Geometry check sheet. Reference: the model listing, model coordinates, mm. Face numbers are marked on the shaded views. A direction names the side the tool comes from. Coordinates: 2 decimals unless noted, no trailing zeros. Write each loop counter-clockwise with the first axis right and the second up, starting at its lowest first coordinate (ties: lowest second). Pieces come first, ordered by that corner, then holes. Notation, with made-up numbers: (33, 33) -> (57, 33) arc R22 ccw to (57, 51) -> close; hole circle Ø3 at (-23.75, 21.5). An arc over 180 degrees is marked (long way). Answer in a Markdown table with one row per item. Add a question column.
Q1. Thickness scan on line 1 (X direction, y = 8.25, z = 4.5); line 2 (Y direction, x = -15.5, z = 5.25); line 3 (Y direction, x = -9.75, z = 5.75). Record the ranges inside material, lowest first.
Q2. Section check D-D, the plane x = -22.75. Record the boundary of the cut face in (y, z).
Q3. Section check A-A, the plane y = 8. Record the boundary of the cut face in (x, z), and give its area (3 significant figures).
Q4. Section check B-B, the plane x = -6. Record the boundary of the cut face in (y, z), and give its area (3 significant figures).
Q5. Tool access check on the marked faces 1, 2 and 3. Record the directions out of +Z, -Z, +X, -X, +Y, -Y that give a thin tool (end or side, any length) a straight path to the whole face; none if there is none.
Q6. Section check C-C, the plane z = 2. Record the boundary of the cut face in (x, y).
Q7. Release check for a two-part mould opening along Z. For the marked faces 4, 5 and 6 record: pulls with the +Z half, pulls with the -Z half, needs draft (parallel to the pull), parting line crosses it, or undercut.
Q8. Gauge pin test, flat ends, axial feed: P1, Ø1.1, axis at x = -23.5, z = 4, coming from the -Y side; P2, Ø0.6, axis at y = 7, z = 4, coming from the -X side; P3, Ø1.6, axis at x = -23.5, y = 7, coming from the +Z side. Record the tip position at first contact, or that the pin passes through.
```python
from build123d import *

# Parameters (mm, degrees)
SKETCH1_W           = 23.5
SKETCH1_H           = 16.2
BOSS_EXTRUDE1_DEPTH = 6.8
FILLET1_R           = 1
SKETCH2_R           = 2.236571794
SKETCH2_W           = 6.565566979
SKETCH2_H           = 4.473143588
SKETCH2_W_2         = 4.671371309
SKETCH2_H_2         = 6.069279627
CUT_EXTRUDE1_DEPTH  = 2
SKETCH3_W           = 4.671371309
SKETCH3_H           = 4.241891526
SKETCH3_W_2         = 6.565566979
SKETCH3_H_2         = 4.084917802
BOSS_EXTRUDE2_DEPTH = 1.8
FILLET2_R           = 1
FILLET3_R           = 2
SKETCH4_R           = 2.01406143
BOSS_EXTRUDE3_DEPTH = 1.8


with BuildPart() as part:
    # Sketch1 → Boss-Extrude1 (new body)
    with BuildSketch(Plane.XY):
        with Locations((-15.007054392, 14.50136894)):
            Rectangle(SKETCH1_W, SKETCH1_H)
    extrude(amount=BOSS_EXTRUDE1_DEPTH)

    # Fillet1
    fillet1_edges = [part.edges().sort_by_distance(p)[0] for p in [
        (-3.257054392, 6.40136894, 3.4),
        (-26.757054392, 6.40136894, 3.4),
    ]]
    fillet(fillet1_edges, radius=FILLET1_R)

    # Sketch2 → Cut-Extrude1 (cut)
    with BuildSketch(Plane.XZ.offset(-6.40136894)):
        with Locations(Location((-15.988556768, 3.515941097, 0), (0, 0, 270))):
            Circle(SKETCH2_R)
        with Locations((-7.901211447, 3.615950214)):
            Rectangle(SKETCH2_W, SKETCH2_H)
        with Locations((-22.557799993, 4.361535506)):
            Rectangle(SKETCH2_W_2, SKETCH2_H_2)
    extrude(amount=-CUT_EXTRUDE1_DEPTH, mode=Mode.SUBTRACT)

    # Sketch3 → Boss-Extrude2 (add)
    with BuildSketch(Plane(origin=(0, 8.40136894, 0), x_dir=(-1, 0, 0), z_dir=(0, -1, 0))):
        with Locations((22.557799993, -3.796232689)):
            Rectangle(SKETCH3_W, SKETCH3_H)
        with Locations((7.901211447, -3.644866315)):
            Rectangle(SKETCH3_W_2, SKETCH3_H_2)
    extrude(amount=BOSS_EXTRUDE2_DEPTH)

    # Fillet2
    fillet2_edges = [part.edges().sort_by_distance(p)[0] for p in [
        (-22.557799992, 6.60136894, 5.917178452),
        (-22.557799992, 6.60136894, 1.675286926),
    ]]
    fillet(fillet2_edges, radius=FILLET2_R)

    # Fillet3
    # the kernel refuses this fillet: 2 mm, written as the material it takes off along each edge
    with BuildSketch(Plane(origin=(-11.183994936, 6.60136894, 5.687325216), x_dir=(0, 1, 0), z_dir=(1, 0, 0))) as fillet3_piece_1:
        with BuildLine():
            CenterArc((2, -1.989974874), FILLET3_R, 95.739170477, 84.260829523)
            Line((0, -1.989974874), (0, 0))
            Line((0, 0), (1.8, 0))
        make_face()
    extrude(amount=6.565566979, mode=Mode.SUBTRACT)
    with BuildSketch(Plane(origin=(-4.618427957, 6.60136894, 1.602407414), x_dir=(0, 0, 1), z_dir=(-1, 0, 0))) as fillet3_piece_2:
        with BuildLine():
            CenterArc((1.989974874, 2), FILLET3_R, 185.739170477, 84.260829523)
            Line((0, 1.8), (0, 0))
            Line((0, 0), (1.989974874, 0))
        make_face()
    extrude(amount=6.565566979, mode=Mode.SUBTRACT)

    # Sketch4 → Boss-Extrude3 (add)
    with BuildSketch(Plane(origin=(0, 8.40136894, 0), x_dir=(-1, 0, 0), z_dir=(0, -1, 0))):
        with Locations(Location((16.007293958, -3.494565095, 0), (0, 0, 90))):
            Circle(SKETCH4_R)
    extrude(amount=BOSS_EXTRUDE3_DEPTH)


solid = part.part
```
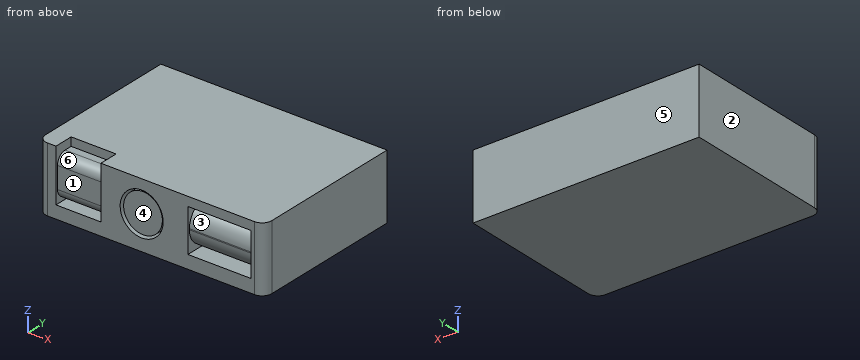
Calculated:
| question | item | result |
|---|---|---|
| 1 | line 1 | x = -26.76 to -18, -17.75 to -14.26, -13.98 to -3.26 |
| 1 | line 2 | y = 6.6 to 22.6 |
| 1 | line 3 | y = 8.4 to 22.6 |
| 2 | outline | (6.4, 0) -> (22.6, 0) -> (22.6, 6.8) -> (8.4, 6.8) -> (8.4, 5.92) -> (7.6, 5.92) arc R1 ccw to (6.6, 4.92) -> (6.6, 2.68) arc R1 ccw to (7.6, 1.68) -> (8.4, 1.68) -> (8.4, 1.33) -> (6.4, 1.33) -> close |
| 3 | outline | (-26.76, 0) -> (-3.26, 0) -> (-3.26, 6.8) -> (-20.22, 6.8) -> (-20.22, 5.92) -> (-24.89, 5.92) -> (-24.89, 6.8) -> (-26.76, 6.8) -> close; circle Ø4.03 at (-16.01, 3.49); hole (-24.89, 1.33) -> (-20.22, 1.33) -> (-20.22, 1.68) -> (-24.89, 1.68) -> close; hole circle Ø4.47 at (-15.99, 3.52); hole (-11.18, 1.38) -> (-4.62, 1.38) -> (-4.62, 1.68) -> (-11.18, 1.68) -> close; hole (-11.18, 5.6) -> (-4.62, 5.6) -> (-4.62, 5.85) -> (-11.18, 5.85) -> close |
| 3 | area | 147 mm² |
| 4 | outline | (6.4, 0) -> (22.6, 0) -> (22.6, 6.8) -> (6.4, 6.8) -> (6.4, 5.85) -> (8.4, 5.85) -> (8.4, 5.69) arc R2 ccw to (6.6, 3.7) -> (6.6, 3.59) arc R2 ccw to (8.4, 1.6) -> (8.4, 1.38) -> (6.4, 1.38) -> close |
| 4 | area | 107 mm² |
| 5 | face 1 | +Z, -Y |
| 5 | face 2 | +Z, -Z, -X, +Y, -Y |
| 5 | face 3 | -Y |
| 6 | outline | (-26.76, 7.4) arc R1 ccw to (-25.76, 6.4) -> (-24.89, 6.4) -> (-24.89, 6.86) -> (-20.22, 6.86) -> (-20.22, 6.4) -> (-17.63, 6.4) -> (-17.63, 8.4) -> (-17.36, 8.4) -> (-17.36, 6.6) -> (-14.66, 6.6) -> (-14.66, 8.4) -> (-14.34, 8.4) -> (-14.34, 6.4) -> (-11.18, 6.4) -> (-11.18, 7.39) -> (-4.62, 7.39) -> (-4.62, 6.4) -> (-4.26, 6.4) arc R1 ccw to (-3.26, 7.4) -> (-3.26, 22.6) -> (-26.76, 22.6) -> close |
| 7 | face 4 | undercut |
| 7 | face 5 | needs draft |
| 7 | face 6 | pulls with the +Z half |
| 8 | P1 | stops at y = 6.6 |
| 8 | P2 | stops at x = -26.75 |
| 8 | P3 | stops at z = 5.92 |
